Source: CAD feature listing. Evaluate the final solid. Frame: model axes, mm. Round coordinates to 2 decimals unless told otherwise and drop trailing zeros. Answer as CSV lines item,"result". Start each with the question number.
```python
from build123d import *

# Parameters (mm, degrees)
UNIVERSAL_PLATE_OUTLINE_W = 72
UNIVERSAL_PLATE_OUTLINE_H = 47
UNIVERSAL_PLATE_OUTLINE_R = 1.5
UNIVERSAL_PLATE_DEPTH     = 1
SKETCH_2_R                = 1.1
CUT_EXTRUDE_1_DEPTH       = 89.743111904


# Read off the part's stored shape, not the designer's step: universal_plate
with BuildPart() as part:
    # universal_plate outline → universal_plate (new body)
    with BuildSketch(Plane.XY):
        with Locations((-42.465454545, 17.942880613)):
            Rectangle(UNIVERSAL_PLATE_OUTLINE_W, UNIVERSAL_PLATE_OUTLINE_H)
        with Locations((-75.965454545, -3.057119387)):
            Circle(UNIVERSAL_PLATE_OUTLINE_R, mode=Mode.SUBTRACT)
        with Locations((-8.965454545, -3.057119387)):
            Circle(UNIVERSAL_PLATE_OUTLINE_R, mode=Mode.SUBTRACT)
        with Locations((-75.965454545, 38.942880613)):
            Circle(UNIVERSAL_PLATE_OUTLINE_R, mode=Mode.SUBTRACT)
        with Locations((-8.965454545, 38.942880613)):
            Circle(UNIVERSAL_PLATE_OUTLINE_R, mode=Mode.SUBTRACT)
    extrude(amount=UNIVERSAL_PLATE_DEPTH)

    # ｽｹｯﾁ2 → ｶｯﾄ - 押し出し1 (cut, through all)
    with BuildSketch(Plane.XY.offset(1)):
        with Locations((-71.465454545, 36.442880613)):
            Circle(SKETCH_2_R)
        with Locations((-55.465454545, 36.442880613)):
            Circle(SKETCH_2_R)
        with Locations((-71.465454545, 20.442880613)):
            Circle(SKETCH_2_R)
        with Locations((-55.465454545, 20.442880613)):
            Circle(SKETCH_2_R)
        with Locations((-50.465454545, 36.442880613)):
            Circle(SKETCH_2_R)
        with Locations((-34.465454545, 36.442880613)):
            Circle(SKETCH_2_R)
        with Locations((-29.465454545, 36.442880613)):
            Circle(SKETCH_2_R)
        with Locations((-13.465454545, 36.442880613)):
            Circle(SKETCH_2_R)
        with Locations((-34.465454545, 20.442880613)):
            Circle(SKETCH_2_R)
        with Locations((-50.465454545, 20.442880613)):
            Circle(SKETCH_2_R)
        with Locations((-13.465454545, 20.442880613)):
            Circle(SKETCH_2_R)
        with Locations((-29.465454545, 20.442880613)):
            Circle(SKETCH_2_R)
        with Locations((-71.465454545, 15.442880613)):
            Circle(SKETCH_2_R)
        with Locations((-55.465454545, 15.442880613)):
            Circle(SKETCH_2_R)
        with Locations((-50.465454545, 15.442880613)):
            Circle(SKETCH_2_R)
        with Locations((-34.465454545, 15.442880613)):
            Circle(SKETCH_2_R)
        with Locations((-29.465454545, 15.442880613)):
            Circle(SKETCH_2_R)
        with Locations((-13.465454545, 15.442880613)):
            Circle(SKETCH_2_R)
        with Locations((-13.465454545, -0.557119387)):
            Circle(SKETCH_2_R)
        with Locations((-29.465454545, -0.557119387)):
            Circle(SKETCH_2_R)
        with Locations((-34.465454545, -0.557119387)):
            Circle(SKETCH_2_R)
        with Locations((-50.465454545, -0.557119387)):
            Circle(SKETCH_2_R)
        with Locations((-55.465454545, -0.557119387)):
            Circle(SKETCH_2_R)
        with Locations((-71.465454545, -0.557119387)):
            Circle(SKETCH_2_R)
    extrude(amount=-CUT_EXTRUDE_1_DEPTH, mode=Mode.SUBTRACT)


solid = part.part
```
1) Section A-A, the plane z = 0.75. Give the number of separate pieces and of enclosed holes in the cut face, and give its area (3 significant figures).
2) Ray query, line 1 along Y through (x, z) = (-34.5, 0.9); line 2 along Y through (x, z) = (-13, 0.65). Return the intervals inside material, ascending.
3) Mould query, pull axis Y, two halves, no side actions, for faces 1 (the cylindrical face through (-30.564, 36.491, 0.507)), 2 (the flat face through (-43, 18, 0)). Classes: pulls with the +Y half, pulls with the -Y half, needs draft (parallel to the pull), parting line crosses it, or undercut.
Findings below:
1,separate pieces,"1"
1,enclosed holes,"28"
1,area,"3,260 mm²"
2,line 1,"-5.56 to -1.66, 0.54 to 14.34, 16.54 to 19.34, 21.54 to 35.34, 37.54 to 41.44"
2,line 2,"-5.56 to -1.55, 0.44 to 14.45, 16.44 to 19.45, 21.44 to 35.45, 37.44 to 41.44"
3,face 1,"undercut"
3,face 2,"needs draft"
